```python
from build123d import *

# Parameters (mm, degrees)
SKETCH1_R            = 2
BOSS_EXTRUDE1_DEPTH  = 60
SKETCH3_R            = 10
SKETCH3_W            = 14
SKETCH3_H            = 7
CUT_EXTRUDE1_DEPTH   = 121.830459736
SKETCH4_W            = 10
SKETCH4_H            = 8.4
CUT_EXTRUDE2_DEPTH   = 87.567892431
SKETCH5_R            = 1.55
CUT_EXTRUDE3_DEPTH   = 88.202350886
FILLET1_R            = 3.5
FILLET1_OF_MIRROR1_R = 3.5


with BuildPart() as part:
    # Sketch1 → Boss-Extrude1 (new, symmetric)
    with BuildSketch(Plane(origin=(0, 0, 0), x_dir=(0, 0, -1), z_dir=(1, 0, 0))):
        Circle(SKETCH1_R)
    extrude(amount=BOSS_EXTRUDE1_DEPTH, both=True)

    # Sketch2 → Revolve2 (revolve)
    with BuildSketch(Plane(origin=(0, 0, 0), x_dir=(1, 0, 0), z_dir=(0, 1, 0)), mode=Mode.PRIVATE) as revolve2_sk:
        Polygon((60, -2), (86, -10), (86, 0), (60, 0), align=None)
    revolve2 = revolve(revolve2_sk.sketch.rotate(Axis((-1000, 0, 0), (1, 0, 0)), 180), axis=Axis((-1000, 0, 0), (1, 0, 0)))

    # Sketch3 → Cut-Extrude1 (cut, through all)
    with BuildSketch(Plane(origin=(60, 0, 0), x_dir=(0, 0, -1), z_dir=(1, 0, 0))):
        Circle(SKETCH3_R)
        Rectangle(SKETCH3_W, SKETCH3_H, mode=Mode.SUBTRACT)
    cut_extrude1 = extrude(amount=CUT_EXTRUDE1_DEPTH, mode=Mode.SUBTRACT)

    # Sketch4 → Cut-Extrude2 (cut, through all)
    with BuildSketch(Plane(origin=(0, 3.5, 0), x_dir=(1, 0, 0), z_dir=(0, 1, 0))):
        with Locations((81, 0)):
            Rectangle(SKETCH4_W, SKETCH4_H)
    cut_extrude2 = extrude(amount=-CUT_EXTRUDE2_DEPTH, mode=Mode.SUBTRACT)

    # Sketch5 → Cut-Extrude3 (cut, through all)
    with BuildSketch(Plane.XY.offset(7)):
        with Locations((82, 0)):
            Circle(SKETCH5_R)
    cut_extrude3 = extrude(amount=-CUT_EXTRUDE3_DEPTH, mode=Mode.SUBTRACT)

    # Fillet1
    fillet1_edges = [part.edges().sort_by_distance(p)[0] for p in [
        (86, -3.5, -5.6),
        (86, 3.5, -5.6),
        (86, -3.5, 5.6),
        (86, 3.5, 5.6),
    ]]
    fillet(fillet1_edges, radius=FILLET1_R - 0.0001)  # a hair under: the kernel refuses the full size

    # Mirror1: Revolve2, Cut-Extrude1, Cut-Extrude2, Cut-Extrude3 across plane
    add(revolve2.mirror(Plane(origin=(0, 0, 0), x_dir=(0, 0, 1), z_dir=(1, 0, 0))))
    add(cut_extrude1.mirror(Plane(origin=(0, 0, 0), x_dir=(0, 0, 1), z_dir=(1, 0, 0))), mode=Mode.SUBTRACT)
    add(cut_extrude2.mirror(Plane(origin=(0, 0, 0), x_dir=(0, 0, 1), z_dir=(1, 0, 0))), mode=Mode.SUBTRACT)
    add(cut_extrude3.mirror(Plane(origin=(0, 0, 0), x_dir=(0, 0, 1), z_dir=(1, 0, 0))), mode=Mode.SUBTRACT)

    # Fillet1 of Mirror1
    fillet1_of_mirror1_edges = [part.edges().sort_by_distance(p)[0] for p in [
        (-86, -3.5, -5.6),
        (-86, 3.5, -5.6),
        (-86, -3.5, 5.6),
        (-86, 3.5, 5.6),
    ]]
    fillet(fillet1_of_mirror1_edges, radius=FILLET1_OF_MIRROR1_R - 0.0001)  # a hair under: the kernel refuses the full size


solid = part.part
```
Source: CAD feature listing. Evaluate the final solid. Frame: model axes, mm. A direction names the side the tool comes from. Round coordinates to 2 decimals unless told otherwise and drop trailing zeros. Loops run counter-clockwise (first coordinate to the right, second up) from the corner with the lowest first, then second, coordinate; pieces in that order, holes last.
(1) Section query A-A (z = 0). Output: boundary loops of the cut face in (x, y) (3 decimals), and give its area (3 significant figures).
From the geometry:
outline: (-76, -3.5) - (-64.875, -3.5) - (-60, -2) - (60, -2) - (64.875, -3.5) - (76, -3.5) - (76, 3.5) - (64.875, 3.5) - (60, 2) - (-60, 2) - (-64.875, 3.5) - (-76, 3.5) - close
area: 689 mm2
(2) Access query for faces 5 (the cylindrical face through (-84.95, -2.5, -5.62)), 6 (the flat face through (-80, 0, 4.2)), 7 (the flat face through (80, 0, -7)), 8 (the flat face through (80, 0, -4.2)), 9 (the conical face through (-65.39, -1.4, -3.38)). Directions: +Z, -Z, +X, -X, +Y, -Y. A direction counts if a zero-diameter tool reaches every point of the face in a straight line with its end or side. Return the directions, or none.
From the geometry:
face 5: +Z, -Z, -X, -Y
face 6: -X, +Y, -Y
face 7: -Z, +X, -X, +Y, -Y
face 8: +X, +Y, -Y
face 9: none
(3) Contact query for flat-ended pins moving along their axis: pin 1 Ø4 at (x, y) = (-11.5, -0.5) entering from +Z; pin 2 Ø1 at (y, z) = (-1.5, -1.5) entering from +X. Output: stop coordinate, or through.
From the geometry:
pin 1: stops at z = 2
pin 2: stops at x = 76
(4) Section query B-B (x = 34). Output: boundary loops of the cut face in (y, z), and give its area (3 significant figures).
From the geometry:
outline: circle Ø4 at (0, 0)
area: 12.6 mm2
(5) Material intervals for probe 1 along Y at (x, z) = (82, -4.85); probe 2 along X at (y, z) = (-1, 0.5); probe 3 along Z at (x, y) = (-50, -1.25), sorted ascending.
From the geometry:
probe 1: y = -3.5 to -1.55, 1.55 to 3.5
probe 2: x = -76 to 76
probe 3: z = -1.56 to 1.56
(6) Pull-direction query (Z, two-part tool) for faces 1 (the cylindrical face through (83.478, 0.466, -5.58)), 2 (the flat face through (76, 0, 0)), 3 (the flat face through (-80, 0, -7)), 4 (the flat face through (-80, 0, -4.2)); classes: +Z half, -Z half, draft (parallel to the pull), parting line (faces both ways), or undercut.
From the geometry:
face 1: draft
face 2: undercut
face 3: -Z half
face 4: undercut
